Model file for the job. Use its own axes, mm. A direction names the side the tool comes from. Round coordinates to 2 decimals unless told otherwise and drop trailing zeros. Loops run counter-clockwise (first coordinate to the right, second up) from the corner with the lowest first, then second, coordinate; pieces in that order, holes last.
Autodesk Inventor part; units mm, degrees
ref_plane "YZ Plane" through (0, 0, 0) normal (1, 0, 0) x (0, 1, 0)
ref_plane "XZ Plane" through (0, 0, 0) normal (0, 1, 0) x (-1, 0, 0)
ref_plane "XY Plane" through (0, 0, 0) normal (0, 0, 1) x (1, 0, 0)
sketch "スケッチ1" plane through (0, 0, 0) normal (1, 0, 0) x (0, 1, 0)
  line L0 (-12.5, 12.5) -> (12.5, 12.5)
  line L1 (12.5, 12.5) -> (12.5, -12.5)
  line L2 (12.5, -12.5) -> (-12.5, -12.5)
  line L3 (-12.5, -12.5) -> (-12.5, 12.5)
  line L4 (-12.5, 12.5) -> (12.5, -12.5) construction
  line L5 (12.5, 12.5) -> (-12.5, -12.5) construction
  point P0 (0, 0)
  dimension "d0" = 25
  dimension "d1" = 25
extrude "押し出し1" add sketch "スケッチ1" along normal blind 75
sketch "スケッチ2" plane through (0, 12.5, 12.5) normal (0, 1, 0) x (1, 0, 0)
  circle A0 centre (10, 12.5) radius 6
  line L0 (0, 0) -> (0, 25)
  line L1 (0, 0) -> (75, 0)
  point P0 (0, 12.5)
  dimension "d4" = 12
  dimension "d5" = 10
  dimension "d6" = 12.5
extrude "押し出し2" cut sketch "スケッチ2" against normal through all
sketch "スケッチ3" plane through (0, 12.5, 12.5) normal (0, 1, 0) x (1, 0, 0)
  circle A0 centre (65, 12.5) radius 4
  line L0 (75, 25) -> (75, 0)
  line L1 (0, 25) -> (75, 25)
  point P0 (0, 12.5)
  dimension "d9" = 10
  dimension "d10" = 8
  dimension "d11" = 12.5
extrude "押し出し3" cut sketch "スケッチ3" against normal through all
sketch "スケッチ4" plane through (75, 0, 0) normal (1, 0, 0) x (0, 0, -1)
  line L0 (-10.2, -10.2) -> (10.2, -10.2)
  line L1 (10.2, -10.2) -> (10.2, 10.2)
  line L2 (10.2, 10.2) -> (-10.2, 10.2)
  line L3 (-10.2, 10.2) -> (-10.2, -10.2)
  line L4 (-10.2, -10.2) -> (10.2, 10.2) construction
  line L5 (10.2, -10.2) -> (-10.2, 10.2) construction
  line L6 (-12.5, 12.5) -> (-12.5, -12.5)
  line L7 (12.5, 12.5) -> (-12.5, 12.5)
  point P0 (0, 0)
  dimension "d14" = 2.3
  dimension "d15" = 2.3
extrude "押し出し4" cut sketch "スケッチ4" against normal through all
sketch "スケッチ5" plane through (0, -12.5, -12.5) normal (0, 0, -1) x (-1, 0, 0)
  line L0 (-75, 2.3) -> (-75, 22.7)
  line L1 (-75, 22.7) -> (-55, 22.7)
  line L2 (-55, 22.7) -> (-55, 2.3)
  line L3 (-55, 2.3) -> (-75, 2.3)
  line L4 (-75, 2.3) -> (-75, 22.7)
  line L5 (-75, 2.3) -> (0, 2.3)
  point P0 (0, 12.5)
  dimension "d18" = 20
extrude "押し出し5" cut sketch "スケッチ5" against normal through all
fillet "フィレット1" radius 7 8 edges at (55, 10.2, 11.35) (55, 10.2, -11.35) (75, 11.35, -12.5) (75, 11.35, 12.5) (75, -11.35, -12.5) (75, -11.35, 12.5) (55, -10.2, 11.35) (55, -10.2, -11.35)
equation "\"d1\" = d0"
properties part number "bracket2" material "鉄、可鍛鉄"
Q1. Tool access for faces 4 (the face through (0, -11, 0)), 5 (the face through (57.1, 8.2, -11.3)): list every direction of +Z, -Z, +X, -X, +Y, -Y with a clear straight run to the whole face (end or side of a thin tool).
Q2. Slice it at B-B on z = 0. Give the cut face in (x, y).
Q3. Slice it at A-A on x = 65. Give the cut face in (y, z), plus the area to 3 significant figures.
Q4. Slice it at D-D on y = -1. Give the cut face in (x, z).
Q5. Slice it at C-C on x = 27.5. Give the cut face in (y, z).
Q6. Probe line 1 (X direction, y = 10.7, z = 0); line 2 (Y direction, x = 10.5, z = 6.5). List the from-to ranges inside material, lowest first.
Q7. Pull direction Z, two halves, no side cores. Call faces 1 (the face through (26, 0, -12.5)), 2 (the face through (75, 11, 0)), 3 (the face through (5.24, 11.37, 3.65)): pulls with the +Z half, pulls with the -Z half, needs draft (parallel to the pull), parting line crosses it, or undercut.
Q8. Flat gauge pin, fed straight in: P1, Ø0.7, axis at y = 0.5, z = -11, coming from the +X side. Where does the tip first touch, or does it go through?
Reply:
1. face 4: +Z, -Z, -X, +Y, -Y
1. face 5: +Z, -Z, +X
2. outline: (0, -12.5) - (4, -12.5) - (4, -10.2) - (0, -10.2) - close; (0, 10.2) - (4, 10.2) - (4, 12.5) - (0, 12.5) - close; (16, -12.5) - (61, -12.5) - (61, -10.2) - (16, -10.2) - close; (16, 10.2) - (61, 10.2) - (61, 12.5) - (16, 12.5) - close; (69, -12.5) - (75, -12.5) - (75, -10.2) - (69, -10.2) - close; (69, 10.2) - (75, 10.2) - (75, 12.5) - (69, 12.5) - close
3. outline: (-12.5, -12.5) - (-10.2, -12.5) - (-10.2, -4) - (-12.5, -4) - close; (-12.5, 4) - (-10.2, 4) - (-10.2, 12.5) - (-12.5, 12.5) - close; (10.2, -12.5) - (12.5, -12.5) - (12.5, -4) - (10.2, -4) - close; (10.2, 4) - (12.5, 4) - (12.5, 12.5) - (10.2, 12.5) - close
3. area: 78.2 mm2
4. outline: (0, -12.5) - (55, -12.5) - (55, -10.2) - (0, -10.2) - close; (0, 10.2) - (55, 10.2) - (55, 12.5) - (0, 12.5) - close
5. outline: (-12.5, -12.5) - (12.5, -12.5) - (12.5, 12.5) - (-12.5, 12.5) - close; hole (-10.2, -10.2) - (10.2, -10.2) - (10.2, 10.2) - (-10.2, 10.2) - close
6. line 1: x = 0 to 4, 16 to 61, 69 to 75
6. line 2: y = -12.5 to -10.2, 10.2 to 12.5
7. face 1: pulls with the -Z half
7. face 2: needs draft
7. face 3: undercut
8. P1: stops at x = 55
